```python
from build123d import *

# Parameters (mm, degrees)
SKETCH2_W           = 79
SKETCH2_H           = 43
BOSS_EXTRUDE1_DEPTH = 2
SKETCH3_W           = 67
SKETCH3_H           = 32
CUT_EXTRUDE1_DEPTH  = 0.7
SKETCH4_W           = 38
SKETCH4_H           = 23
CUT_EXTRUDE2_DEPTH  = 0.7
SKETCH7_R           = 6
BOSS_EXTRUDE2_DEPTH = 13
SKETCH8_W           = 10
SKETCH8_H           = 7
BOSS_EXTRUDE3_DEPTH = 1
SKETCH9_W           = 7
SKETCH9_H           = 5
BOSS_EXTRUDE4_DEPTH = 1
SKETCH10_W          = 71
SKETCH10_H          = 39
BOSS_EXTRUDE5_DEPTH = 33
SKETCH11_W          = 20
SKETCH11_H          = 18
CUT_EXTRUDE3_DEPTH  = 10
BOSS_EXTRUDE6_DEPTH = 2.5
BOSS_EXTRUDE7_DEPTH = 2.5


with BuildPart() as part:
    # Sketch2 → Boss-Extrude1 (new body)
    with BuildSketch(Plane(origin=(0, 0, 0), x_dir=(1, 0, 0), z_dir=(0, 1, 0))):
        with Locations((39.5, 21.5)):
            Rectangle(SKETCH2_W, SKETCH2_H)
    extrude(amount=BOSS_EXTRUDE1_DEPTH)

    # Sketch3 → Cut-Extrude1 (cut)
    with BuildSketch(Plane(origin=(0, 2, 0), x_dir=(1, 0, 0), z_dir=(0, 1, 0))):
        with Locations((39.5, 21.5)):
            Rectangle(SKETCH3_W, SKETCH3_H)
    extrude(amount=-CUT_EXTRUDE1_DEPTH, mode=Mode.SUBTRACT)

    # Sketch4 → Cut-Extrude2 (cut)
    with BuildSketch(Plane(origin=(0, 1.3, 0), x_dir=(1, 0, 0), z_dir=(0, 1, 0))):
        with Locations((36, 22)):
            Rectangle(SKETCH4_W, SKETCH4_H)
    extrude(amount=-CUT_EXTRUDE2_DEPTH, mode=Mode.SUBTRACT)

    # Sketch7 → Boss-Extrude2 (add)
    with BuildSketch(Plane(origin=(0, 1.3, 0), x_dir=(1, 0, 0), z_dir=(0, 1, 0))):
        with Locations((65.5, 27.5)):
            Circle(SKETCH7_R)
    extrude(amount=BOSS_EXTRUDE2_DEPTH)

    # Sketch8 → Boss-Extrude3 (add)
    with BuildSketch(Plane(origin=(0, 1.3, 0), x_dir=(1, 0, 0), z_dir=(0, 1, 0))):
        with Locations((65.5, 14)):
            Rectangle(SKETCH8_W, SKETCH8_H)
    extrude(amount=BOSS_EXTRUDE3_DEPTH)

    # Sketch9 → Boss-Extrude4 (add)
    with BuildSketch(Plane(origin=(0, 1.3, 0), x_dir=(1, 0, 0), z_dir=(0, 1, 0))):
        with Locations((11.5, 14)):
            Rectangle(SKETCH9_W, SKETCH9_H)
        with Locations((11.5, 29)):
            Rectangle(SKETCH9_W, SKETCH9_H)
    extrude(amount=BOSS_EXTRUDE4_DEPTH)

    # Sketch10 → Boss-Extrude5 (add)
    with BuildSketch(Plane.XZ):
        with Locations((39.5, -21.5)):
            Rectangle(SKETCH10_W, SKETCH10_H)
    extrude(amount=BOSS_EXTRUDE5_DEPTH)

    # Sketch11 → Cut-Extrude3 (cut)
    with BuildSketch(Plane(origin=(0, -33, 0), x_dir=(-1, 0, 0), z_dir=(0, -1, 0))):
        with Locations((-39.5, 2)):
            Rectangle(SKETCH11_W, SKETCH11_H)
    extrude(amount=-CUT_EXTRUDE3_DEPTH, mode=Mode.SUBTRACT)

    # Sketch12 → Boss-Extrude6 (add)
    with BuildSketch(Plane.ZY.offset(-4)):
        Polygon((-21.5, 0), (-27.5, 0), (-27.5, -11), (-21.5, -11), (-15.5, -11), (-15.5, 0), align=None)
    extrude(amount=BOSS_EXTRUDE6_DEPTH)

    # Sketch13 → Boss-Extrude7 (add)
    with BuildSketch(Plane(origin=(75, 0, 0), x_dir=(0, 0, -1), z_dir=(1, 0, 0))):
        Polygon((21.5, 0), (15.5, 0), (15.5, -11), (21.5, -11), (27.5, -11), (27.5, 0), align=None)
    extrude(amount=BOSS_EXTRUDE7_DEPTH)


solid = part.part
```
Read the model definition and answer for the solid it produces. Units are mm, in the model's axes. A direction names the side the tool comes from. Coordinates: 2 decimals unless noted, no trailing zeros. Loops run counter-clockwise (first coordinate to the right, second up) from the corner with the lowest first, then second, coordinate; pieces in that order, holes last.
(1) The part is cut by section D-D (y = -30). Determine the outline of the cut face in (x, z).
Solution:
outline: (4, -41) - (75, -41) - (75, -2) - (49.5, -2) - (49.5, -11) - (29.5, -11) - (29.5, -2) - (4, -2) - close
(2) The part is cut by section A-A (x = 26). Determine the outline of the cut face in (y, z).
Solution:
outline: (-33, -41) - (0, -41) - (0, -43) - (2, -43) - (2, -37.5) - (1.3, -37.5) - (1.3, -33.5) - (0.6, -33.5) - (0.6, -10.5) - (1.3, -10.5) - (1.3, -5.5) - (2, -5.5) - (2, 0) - (0, 0) - (0, -2) - (-33, -2) - close
(3) Consider line 1 along Y through (x, z) = (48.5, -28.5); line 2 along Y through (x, z) = (72, -30); line 3 along X through (y, z) = (-21, -30). Determine where each line is inside the solid, lowest interval first.
Solution:
line 1: y = -33 to 0.6
line 2: y = -33 to 1.3
line 3: x = 4 to 75
(4) The part is cut by section B-B (z = -13). Determine the outline of the cut face in (x, y), and give its area (3 significant figures).
Solution:
outline: (0, 0) - (4, 0) - (4, -33) - (75, -33) - (75, 0) - (79, 0) - (79, 2) - (73, 2) - (73, 1.3) - (70.5, 1.3) - (70.5, 2.3) - (60.5, 2.3) - (60.5, 1.3) - (55, 1.3) - (55, 0.6) - (17, 0.6) - (17, 1.3) - (15, 1.3) - (15, 2.3) - (8, 2.3) - (8, 1.3) - (6, 1.3) - (6, 2) - (0, 2) - close
area: 2,440 mm2
(5) The part is cut by section C-C (y = -7). Determine the outline of the cut face in (x, z).
Solution:
outline: (1.5, -27.5) - (4, -27.5) - (4, -41) - (75, -41) - (75, -27.5) - (77.5, -27.5) - (77.5, -15.5) - (75, -15.5) - (75, -2) - (4, -2) - (4, -15.5) - (1.5, -15.5) - close
(6) Flat-ended cylindrical pins translate along their axes: pin 1 Ø10 at (x, y) = (45, -16) entering from +Z; pin 2 Ø0.5 at (x, y) = (64.5, 1.5) entering from +Z; pin 3 Ø3 at (y, z) = (-6.5, -18.5) entering from +X; pin 4 Ø3 at (y, z) = (-28, -36.5) entering from +X. Find the tip coordinate at first contact, or state that the pin passes through.
Solution:
pin 1: stops at z = -2
pin 2: stops at z = 0
pin 3: stops at x = 77.5
pin 4: stops at x = 75
(7) A tool of negligible diameter and unlimited length cuts with its end or side. For faces 5 (the face through (49.5, -28, -6)), 6 (the face through (76, -6, -27.5)), 7 (the face through (3, -5, -27.5)), 8 (the face through (76, -5, -15.5)), from which of +Z, -Z, +X, -X, +Y, -Y can it reach the whole face along a straight path? Write none if from no direction.
Solution:
face 5: +Z, -Y
face 6: -Z, +X, -Y
face 7: -Z, -X, -Y
face 8: +Z, +X, -Y
(8) The mould has two halves that part along X. Classify faces 1 (the face through (0, 1, -21)), 2 (the face through (29.5, -28, -6)), 3 (the face through (77.5, -5, -21)), 4 (the face through (39, -33, -21)): released by +X, released by -X, zero draft, split by the parting line, or undercut.
Solution:
face 1: released by -X
face 2: undercut
face 3: released by +X
face 4: zero draft
